Source: three-view drawing plus pictorial views. Frame: mm from the lowest corner of the part. Give positions to 0.01 mm unless a question says otherwise; leave off trailing zeros. Order: outer loops, then holes, each group sorted by start corner. A loop starts at its lowest first (then second) coordinate and runs counter-clockwise, first axis right, second up. Notation, with made-up numbers: (78.25, 45) - (134.25, 45) arc R16 ccw to (134.25, 51) - close; hole circle Ø10 at (89.25, -33.75). An arc over 180 degrees is marked (long way). Use one line per item in the form item = value.
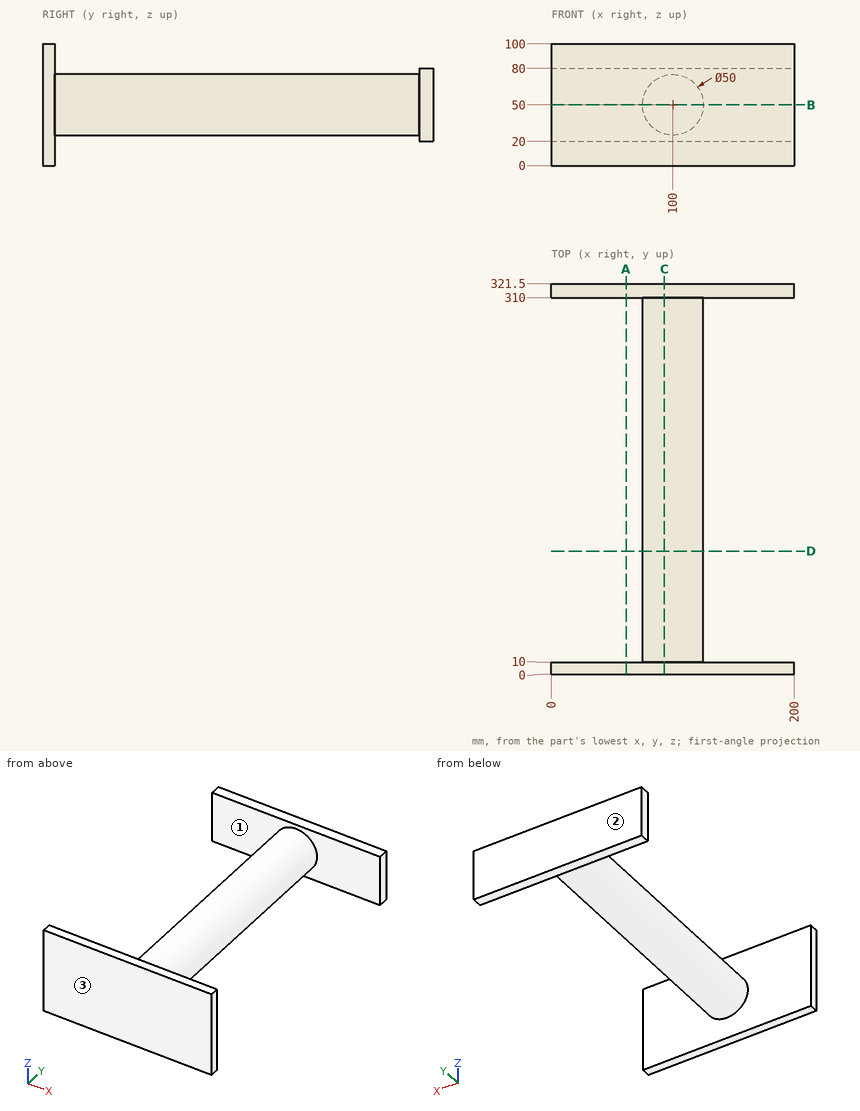
(1) Cut plane D-D on y = 101.5. Output: boundary loops of the cut face in (x, z).
Computed values:
outline = circle Ø50 at (100, 50)
(2) Contact query for flat-ended pins moving along their axis: pin 1 Ø3.5 at (x, y) = (65.5, 318) entering from +Z; pin 2 Ø12.5 at (x, y) = (57, 314.5) entering from -Z; pin 3 Ø3 at (y, z) = (37, 71.5) entering from -X. Output: stop coordinate, or through.
Computed values:
pin_1 = 80
pin_2 = 20
pin_3 = 85
(3) Cut plane C-C on x = 93. Output: boundary loops of the cut face in (y, z), plus the area to 3 significant figures.
Computed values:
outline = (0, 0) - (10, 0) - (10, 26) - (310, 26) - (310, 20) - (321.5, 20) - (321.5, 80) - (310, 80) - (310, 74) - (10, 74) - (10, 100) - (0, 100) - close
area = 16,100 mm²
(4) Ray query, line 1 along Y through (x, z) = (173.5, 78.5); line 2 along Y through (x, z) = (100, 18); line 3 along Z through (x, y) = (105, 235). Return the intervals inside material, ascending.
Computed values:
line_1 = 0 to 10, 310 to 321.5
line_2 = 0 to 10
line_3 = 25.51 to 74.49
(5) Pull-direction query (Y, two-part tool) for the marked faces 1, 2 and 3; classes: released by +Y, released by -Y, zero draft, split by the parting line, or undercut.
Computed values:
face_1 = undercut
face_2 = released by +Y
face_3 = released by -Y
(6) Cut plane A-A on x = 61.5. Output: boundary loops of the cut face in (y, z), plus the area to 3 significant figures.
Computed values:
outline = (0, 0) - (10, 0) - (10, 100) - (0, 100) - close; (310, 20) - (321.5, 20) - (321.5, 80) - (310, 80) - close
area = 1,690 mm²
(7) Cut plane B-B on z = 50. Output: boundary loops of the cut face in (x, y), plus the area to 3 significant figures.
Computed values:
outline = (0, 0) - (200, 0) - (200, 10) - (125, 10) - (125, 310) - (200, 310) - (200, 321.5) - (0, 321.5) - (0, 310) - (75, 310) - (75, 10) - (0, 10) - close
area = 19,300 mm²
